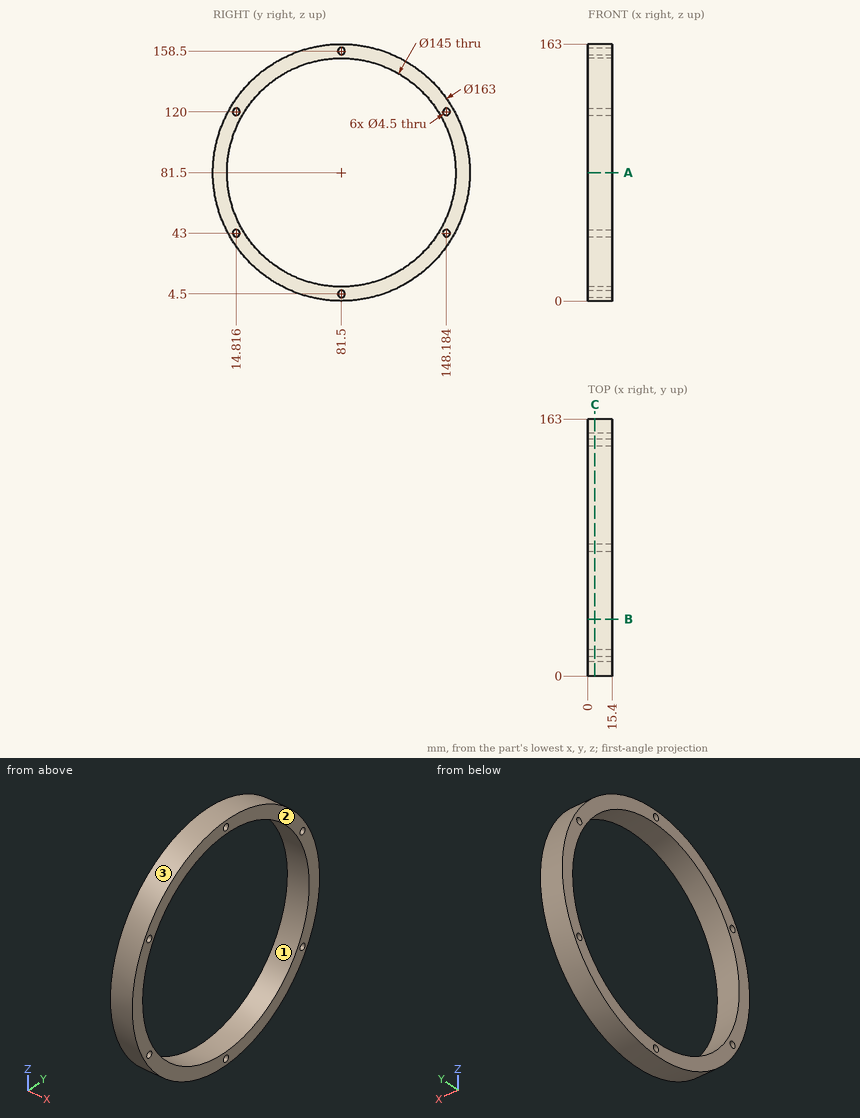
Can you work these out from the drawing? Everything is in mm from the part's minimum corner. Round coordinates to 2 decimals unless told otherwise and drop trailing zeros. Loops run counter-clockwise (first coordinate to the right, second up) from the corner with the lowest first, then second, coordinate; pieces in that order, holes last. Notation, with made-up numbers: (27.5, -35.5) - (42.5, -35.5) arc R27 cw to (42.5, 1.5) - close; hole circle Ø4 at (37.5, 55.5). An arc over 180 degrees is marked (long way). One line per question, with ' | ' between items. Start each with the question number.
Q1. We'd pull the mould along Y, two halves only. Please class the marked faces 1, 2 and 3: +Y half, -Y half, draft (parallel to the pull), parting line (faces both ways), or undercut.
Q2. I want a section at C-C (x = 4.5). Write out the boundary of the cut face in (y, z) (3 decimals), then the cut area to 3 significant figures.
Q3. I want a section at A-A (z = 81.5). Write out the boundary of the cut face in (x, y), then the cut area to 3 significant figures.
Q4. Will these pins go through, and if not, where does the flat tip stop? pin 1 (8 mm diameter, centred on x = 10.5, y = 70.5, fed in from -Z); pin 2 (5 mm diameter, centred on y = 148.18, z = 43, fed in from +X); pin 3 (3 mm diameter, centred on x = 2, z = 16.5, fed in from +Y); pin 4 (1.5 mm diameter, centred on x = 10.5, z = 128, fed in from -Y).
Q5. I want a section at B-B (y = 36). Write out the boundary of the cut face in (x, z).
Q6. Please list where these lines run through material, in increasing order: line 1 (Z direction, x = 1.5, y = 15); line 2 (Y direction, x = 1, z = 119); line 3 (Y direction, x = 6.5, z = 81.5). Write a range as [from, to].
Response values:
1) face 1: undercut | face 2: draft | face 3: parting line
2) outline: circle Ø163 at (81.5, 81.5); hole circle Ø145 at (81.5, 81.5); hole circle Ø4.5 at (14.816, 43); hole circle Ø4.5 at (14.816, 120); hole circle Ø4.5 at (81.5, 4.5); hole circle Ø4.5 at (81.5, 158.5); hole circle Ø4.5 at (148.184, 43); hole circle Ø4.5 at (148.184, 120) | area: 4,260 mm²
3) outline: (0, 0) - (15.4, 0) - (15.4, 9) - (0, 9) - close; (0, 154) - (15.4, 154) - (15.4, 163) - (0, 163) - close | area: 277 mm²
4) pin 1: stops at z = 0.3 | pin 2: stops at x = 15.4 | pin 3: stops at y = 132.59 | pin 4: stops at y = 14.05
5) outline: (0, 13.88) - (15.4, 13.88) - (15.4, 25.06) - (0, 25.06) - close; (0, 137.94) - (15.4, 137.94) - (15.4, 149.12) - (0, 149.12) - close
6) line 1: z = [34.38, 40.76], [45.24, 52.62], [110.38, 117.76], [122.24, 128.62] | line 2: y = [9.14, 12.8], [16.83, 19.45], [143.55, 146.17], [150.2, 153.86] | line 3: y = [0, 9], [154, 163]
